Here's how the part is built. I have some questions about the finished solid (model axes, mm). A direction names the side the tool comes from. Coordinates: 2 decimals unless noted, no trailing zeros. Write each loop counter-clockwise with the first axis right and the second up, starting at its lowest first coordinate (ties: lowest second). Pieces come first, ordered by that corner, then holes. Notation, with made-up numbers: (27.5, -39) - (53.5, -39) arc R12 cw to (53.5, -31) - close; hole circle Ø8 at (47.5, -34). An arc over 180 degrees is marked (long way). Answer in a Markdown table with one row per item. Add a question column.
Item 1: If I drill on probe 1 along X at (y, z) = (4.25, 0); probe 2 along Y at (x, z) = (11.5, -26.5); probe 3 along Z at (x, y) = (-3, 8), over which ranges is the centre line in solid material (lowest first)? Write a range as from..to.
Item 2: Imagine slicing it at D-D (x = -25). Please give me the cut outline in (y, z).
Item 3: We'd pull the mould along Z, two halves only. Please class faces 1 (the face through (-0.488, 7.028, -22.804)), 2 (the face through (-22.854, 7.028, -0.676)), 3 (the face through (-20, 5, 6)), 4 (the face through (-20.013, 2.465, -4.444)): +Z half, -Z half, draft (parallel to the pull), parting line (faces both ways), or undercut.
Item 4: I'm going to push flat-ended pins straight in: pin 1 (4 mm diameter, centred on x = -5.5, z = 1, fed in from -Y); pin 2 (1.5 mm diameter, centred on x = -7.5, z = -20.5, fed in from -Y); pin 3 (5 mm diameter, centred on x = -20, y = 7.5, fed in from +Z); pin 4 (1 mm diameter, centred on y = 5, z = 7, fed in from -X). Where does each tip first touch, or does it pass through?
Item 5: Which directions (+Z, -Z, +X, -X, +Y, -Y) give clear straight access to the entire face, cutting with the end or side of a thin tool? Please do faces 5 (the face through (2.5, 5, 7)), 6 (the face through (-6, 9, 6)).
Item 6: Imagine slicing it at B-B (y = 6.25). Please give me the cut outline in (x, z).
Item 7: Imagine slicing it at C-C (y = 2.25). Please give me the cut outline in (x, z), plus the area to 3 significant figures.
Item 8: Imagine slicing it at A-A (z = 0). Please give me the cut outline in (x, y), plus the area to 3 significant figures.
from build123d import *

# Parameters (mm, degrees)
SKIZZE1_R                            = 20.5
SKIZZE1_R_2                          = 7
AUFSATZ_LINEAR_AUSTRAGEN1_DEPTH      = 5
SKIZZE3_R                            = 30
SKIZZE3_R_2                          = 7
AUFSATZ_LINEAR_AUSTRAGEN2_DEPTH      = 4
DURCHGANGSLOCH_F_R_M41_D             = 4.5
SCHNITT_LINEAR_AUSTRAGEN1_DEPTH      = 44.370496884
SCHNITT_LINEAR_AUSTRAGEN1_DEPTH_BACK = 44.370496884


with BuildPart() as part:
    # Skizze1 → Aufsatz-Linear austragen1 (new body)
    with BuildSketch(Plane(origin=(0, 0, 0), x_dir=(1, 0, 0), z_dir=(0, 1, 0))):
        with Locations(Location((0, 0, 0), (0, 0, 270))):
            Circle(SKIZZE1_R)
        with Locations(Location((0, 0, 0), (0, 0, 270))):
            Circle(SKIZZE1_R_2, mode=Mode.SUBTRACT)
    extrude(amount=AUFSATZ_LINEAR_AUSTRAGEN1_DEPTH)

    # Skizze3 → Aufsatz-Linear austragen2 (add)
    with BuildSketch(Plane(origin=(0, 5, 0), x_dir=(1, 0, 0), z_dir=(0, 1, 0))):
        with Locations(Location((0, 0, 0), (0, 0, 270))):
            Circle(SKIZZE3_R)
        with Locations(Location((0, 0, 0), (0, 0, 270))):
            Circle(SKIZZE3_R_2, mode=Mode.SUBTRACT)
    extrude(amount=AUFSATZ_LINEAR_AUSTRAGEN2_DEPTH)

    # Durchgangsloch für M41 (through all)
    with Locations(Plane(origin=(0, 5, 0), x_dir=(-1, 0, 0), z_dir=(0, -1, 0))):
        with Locations((0, 25), (-25, 0), (0, -25), (25, 0)):
            Hole(DURCHGANGSLOCH_F_R_M41_D / 2)

    # Skizze6 → Schnitt-Linear austragen1 (cut, two sides: drawn at the far end of the back side and taken through both)
    with BuildSketch(Plane.XZ.offset(-SCHNITT_LINEAR_AUSTRAGEN1_DEPTH_BACK)):
        with BuildLine():
            Line((2.5, 7.838348415), (-2.5, 7.838348415))
            Line((-2.5, 7.838348415), (-2.5, 6.538348415))
            ThreePointArc((-2.5, 6.538348415), (0, 7), (2.5, 6.538348415))
            Line((2.5, 6.538348415), (2.5, 7.838348415))
        make_face()
    extrude(amount=SCHNITT_LINEAR_AUSTRAGEN1_DEPTH + SCHNITT_LINEAR_AUSTRAGEN1_DEPTH_BACK, mode=Mode.SUBTRACT)


solid = part.part
Here are the results:
| question | item | result |
|---|---|---|
| 1 | probe 1 | x = -20.5..-7, 7..20.5 |
| 1 | probe 2 | y = 5..9 |
| 1 | probe 3 | z = -29.85..-6.32, 6.32..29.85 |
| 2 | outline | (5, -16.58) - (9, -16.58) - (9, -2.25) - (5, -2.25) - close; (5, 2.25) - (9, 2.25) - (9, 16.58) - (5, 16.58) - close |
| 3 | face 1 | undercut |
| 3 | face 2 | undercut |
| 3 | face 3 | draft |
| 3 | face 4 | parting line |
| 4 | pin 1 | stops at y = 0 |
| 4 | pin 2 | stops at y = 5 |
| 4 | pin 3 | stops at z = 24.37 |
| 4 | pin 4 | stops at x = -29.29 |
| 5 | face 5 | +Y, -Y |
| 5 | face 6 | +Z, -Z, +X, -X, +Y |
| 6 | outline | circle Ø60 at (0, 0); hole circle Ø4.5 at (-25, 0); hole (-2.5, 6.54) arc R7 ccw (long way) to (2.5, 6.54) - (2.5, 7.84) - (-2.5, 7.84) - close; hole circle Ø4.5 at (0, -25); hole circle Ø4.5 at (0, 25); hole circle Ø4.5 at (25, 0) |
| 7 | outline | circle Ø41 at (0, 0); hole (-2.5, 6.54) arc R7 ccw (long way) to (2.5, 6.54) - (2.5, 7.84) - (-2.5, 7.84) - close |
| 7 | area | 1,160 mm2 |
| 8 | outline | (-30, 5) - (-27.25, 5) - (-27.25, 9) - (-30, 9) - close; (-22.75, 5) - (-20.5, 5) - (-20.5, 0) - (-7, 0) - (-7, 9) - (-22.75, 9) - close; (7, 0) - (20.5, 0) - (20.5, 5) - (22.75, 5) - (22.75, 9) - (7, 9) - close; (27.25, 5) - (30, 5) - (30, 9) - (27.25, 9) - close |
| 8 | area | 283 mm2 |
